For this review, take the finished solid that the model builds, in its own axes (mm). Face numbers are marked on the shaded views. A direction names the side the tool comes from. Give positions to 0.01 mm unless a question says otherwise; leave off trailing zeros. Loops run counter-clockwise (first coordinate to the right, second up) from the corner with the lowest first, then second, coordinate; pieces in that order, holes last. Notation, with made-up numbers: (22, -20) -> (39, -20) arc R30 cw to (39, 17) -> close; hole circle Ø7 at (19, -31). An arc over 180 degrees is marked (long way). Answer as CSV lines item,"result". Start each with the question number.
Item 1: Add section D-D on y = -4. State how many separate pieces and enclosed holes the cut face has, plus the area to 3 significant figures.
Item 2: For L1, parallel to X at y = -6.75, z = -5; L2, parallel to X at y = -6.25, z = -0.75; L3, parallel to Y at x = 24.5, z = 1.5, list the stretches that pass through material, from the lowest coordinate up. Write a range as from..to.
Item 3: Clearance check with flat-ended pins moving along their axes: P1, Ø1.5, axis at x = 28.5, y = -1, coming from the -Z side; P2, Ø1, axis at y = 0, z = -7.5, coming from the -X side; P3, Ø3.5, axis at x = 31.5, y = -2, coming from the -Z side. State where each tip first meets the part, or that it passes through.
Item 4: The part is to be moulded in two halves that separate along Y. For the marked faces 1, 2, 3 and 4, say which applies: +Y half, -Y half, draft (parallel to the pull), parting line (faces both ways), or undercut.
Item 5: Machinability: for the marked faces 5, 6 and 7, which of the approach directions +Z, -Z, +X, -X, +Y, -Y give a long, thin tool a straight path to every point of the face, cutting with its end or side? Answer none if there is none.
Item 6: Add section A-A on x = 29. State the section outline as (y, z) points.
Item 7: Add section C-C on z = -7. State the section outline as (x, y) points.
Item 8: Add section B-B on y = -8.5. State the section outline as (x, z) points, plus the area to 3 significant figures.
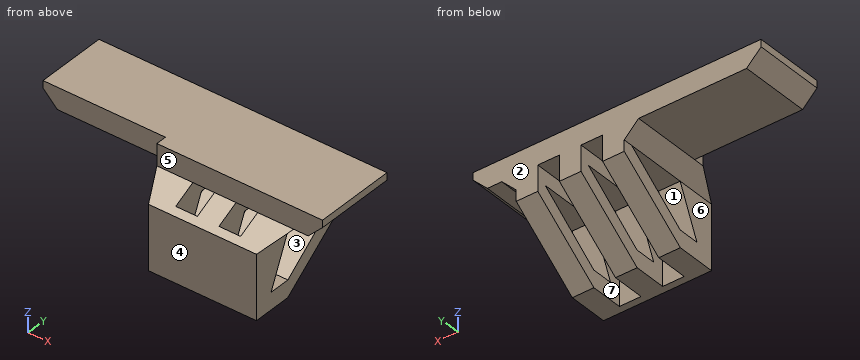
Autodesk Inventor part; units mm, degrees
ref_plane "YZ Plane" through (0, 0, 0) normal (1, 0, 0) x (0, 1, 0)
ref_plane "XZ Plane" through (0, 0, 0) normal (0, 1, 0) x (-1, 0, 0)
ref_plane "XY Plane" through (0, 0, 0) normal (0, 0, 1) x (1, 0, 0)
sketch "Sketch1" plane through (0, 0, 0) normal (0, 0, 1) x (1, 0, 0)
  line L0 (0, 0) -> (5, 0)
  line L1 (5, 0) -> (19, 0)
  line L2 (19, 0) -> (33, 0)
  line L3 (33, 0) -> (28, 0)
  circle A0 centre (5, 0) radius 5
  circle A1 centre (19, 0) radius 5
  circle A2 centre (33, 0) radius 5
  line L4 (0, 0) -> (-1, 0)
  line L5 (38, 0) -> (39, 0)
  line L6 (33, -5) -> (33, -6)
  line L7 (-1, 6) -> (39, 6)
  line L8 (39, 6) -> (39, -6)
  line L9 (39, -6) -> (-1, -6)
  line L10 (-1, -6) -> (-1, 6)
  dimension "d0" = 5
  dimension "d1" = 14
  dimension "d2" = 14
  dimension "d3" = 5
  dimension "d4" = 10
  dimension "d5" = 10
  dimension "d6" = 10
  dimension "d9" = 1
  dimension "d10" = 1
  dimension "d11" = 1
extrude "Extrusion1" add sketch "Sketch1" along normal blind 3
sketch "Sketch2" plane through (-1, 6, 0) normal (0, 1, 0) x (1, 0, 0)
  line L0 (0, -3) -> (40, -3)
  line L1 (19, 2) -> (19, 12)
  line L2 (19, 12) -> (34, 12)
  line L3 (34, 12) -> (34, 2)
  line L4 (34, 0) -> (19, 0)
  line L5 (40, 0) -> (36, 0)
  line L6 (36, 0) -> (34, 2)
  line L7 (0, 0) -> (40, 0)
  line L8 (17, 0) -> (0, 0)
  line L9 (19, 2) -> (17, 0)
  line L10 (36, 0) -> (17, 0)
  point P0 (1, 0)
  dimension "d16" = 12
  dimension "d17" = 2
  dimension "d19" = 2
  dimension "d20" = 2
extrude "Extrusion2" add sketch "Sketch2" against normal blind 16
sketch "Sketch3" plane through (-1, 6, 3) normal (0, 1, 0) x (1, 0, 0)
  line L0 (34, 5) -> (34, 15)
  line L1 (34, 5) -> (34, -8.5215)
  line L2 (34, -8.5215) -> (31, -8.5215)
  line L3 (31, -8.5215) -> (28, -8.5215)
  line L4 (28, -8.5215) -> (25, -8.5215)
  line L5 (25, -8.5215) -> (22, -8.5215)
  line L6 (22, -8.5215) -> (19, -8.5215)
  line L7 (34, 5) -> (34, 3)
  line L8 (17, 3) -> (36, 3)
  line L9 (31, 3) -> (31, 15)
  line L10 (34, 15) -> (19, 15)
  line L11 (31, 15) -> (34, 15)
  line L12 (34, 15) -> (34, 5)
  line L13 (34, 3) -> (31, 3)
  line L14 (31, 3) -> (28, 3)
  line L15 (28, 3) -> (28, 15)
  line L16 (28, 15) -> (31, 15)
  line L17 (28, 3) -> (25, 3)
  line L18 (25, 3) -> (25, 15)
  line L19 (25, 15) -> (28, 15)
  line L20 (25, 3) -> (22, 3)
  line L21 (22, 3) -> (22, 15)
  line L22 (22, 15) -> (25, 15)
  line L23 (22, 3) -> (19, 3)
  line L24 (19, 15) -> (19, 5)
  line L25 (19, 3) -> (19, 15)
  line L26 (19, 15) -> (22, 15)
  point P0 (1, 3)
  dimension "d27" = 3
  dimension "d28" = 3
  dimension "d29" = 3
  dimension "d30" = 3
  dimension "d31" = 3
extrude "Extrusion3" cut sketch "Sketch3" against normal blind 15 contours L9 L8 L15 L10 | L18 L8 L21 L10
sketch "Sketch4" plane through (39, -6, 0) normal (1, 0, 0) x (0, 0, -1)
  line L0 (2, 12) -> (2, -4)
  line L1 (0, 0) -> (2, -4)
  line L2 (2, -4) -> (2, 0)
  line L3 (0, 0) -> (2, 0)
  line L4 (2, 12) -> (2, 10)
  line L5 (12, -3) -> (2, 10)
  line L6 (2, 0) -> (2, 1.5)
  line L7 (2, 10) -> (2, 1.5)
  line L8 (2, 1.5) -> (12, -3)
  line L9 (2, 12) -> (12, 12)
  line L10 (12, 12) -> (12, -4)
  line L11 (12, -3) -> (12, -1)
  line L12 (12, -1) -> (12, 0)
  line L13 (12, 0) -> (3, 12)
  line L14 (2, 12) -> (3, 12)
  line L15 (3, 12) -> (12, 12)
  line L16 (12, 12) -> (12, 0)
  line L17 (0, 0) -> (0, -3)
  line L18 (0, 0) -> (0, -4)
  line L19 (0, 0) -> (0, -4)
  line L20 (2, -4) -> (0, -4)
  line L21 (0, -4) -> (2, -4)
  line L22 (8.5385, 1.5) -> (8.5385, -1.4423)
  point P0 (0, 6)
  dimension "d34" = 2
  dimension "d35" = 1.5
  dimension "d37" = 2
  dimension "d38" = 1
extrude "Extrusion5" cut sketch "Sketch4" against normal blind 25 contours L5 L22 L8 L0 | L9 L10 L13 | L20 L18 L17 L1
chamfer "Chamfer1" distance 2 angle 45 1 edges at (-1, 0, 0)
chamfer "Chamfer2" distance 2 angle 45 1 edges at (39, 0, 0)
sketch "Sketch5" plane through (33, 6, -2) normal (1, 0, 0) x (0, 0, -1)
  line L0 (10, -16) -> (0, -16)
  line L1 (10, -16) -> (8.9, -16)
  line L2 (8.9, -16) -> (8.9, -9)
  line L3 (8.9, -9) -> (10, -9)
  line L4 (10, -9) -> (10, -16)
  point P0 (-2, -6)
  dimension "d49" = 1.1
  dimension "d50" = 7
extrude "Extrusion6" cut sketch "Sketch5" against normal blind 15
sketch "Sketch6" plane through (0, 0, 0) normal (0, 0, -1) x (-1, 0, 0)
  line L0 (-1, -6) -> (-16, -6)
  line L1 (1, 6) -> (1, -6)
  line L2 (-16, -6) -> (1, -6)
  line L3 (1, -6) -> (1, -4.5)
  line L4 (1, -4.5) -> (-16, -4.5)
  line L5 (-16, -4.5) -> (-16, -6)
  point P0 (0, 0)
  dimension "d53" = 1.5
extrude "Extrusion7" cut sketch "Sketch6" against normal blind 10
sketch "Sketch7" plane through (0, 0, 3) normal (0, 0, 1) x (1, 0, 0)
  line L0 (39, 6) -> (-1, 6)
  line L1 (39, -6) -> (39, 6)
  line L2 (-1, 6) -> (39, 6)
  line L3 (39, 6) -> (39, 5.3)
  line L4 (39, 5.3) -> (-1, 5.3)
  line L5 (-1, 5.3) -> (-1, 6)
  point P0 (0, 0)
  dimension "d56" = 0.7
extrude "Extrusion8" cut sketch "Sketch7" against normal blind 10
equation "\"d20\" = d19"
properties part number "StandBtn"
Computed values:
1,separate pieces,"4"
1,enclosed holes,"0"
1,area,"159 mm²"
2,L1,"18..21, 24..27, 30..33"
2,L2,"16.75..21, 24..27, 30..34.25"
2,L3,"-6..5.3"
3,P1,"z = 0"
3,P2,"x = 18"
3,P3,"z = -10.31"
4,face 1,"undercut"
4,face 2,"+Y half"
4,face 3,"undercut"
4,face 4,"-Y half"
5,face 5,"+Z, +X, -X, -Y"
5,face 6,"-Z, -X, +Y, -Y"
5,face 7,"-Z, +Y"
6,outline,"(-10, -10.9) -> (-9, -10.9) -> (-9, -1.5) -> (-10, -2) -> close; (-6, 0) -> (5.3, 0) -> (5.3, 3) -> (-6, 3) -> close"
7,outline,"(18, -10) -> (33, -10) -> (33, -6.75) -> (30, -6.75) -> (30, -9) -> (27, -9) -> (27, -6.75) -> (24, -6.75) -> (24, -9) -> (21, -9) -> (21, -6.75) -> (18, -6.75) -> close; (18, -2.5) -> (21, -2.5) -> (21, 0.67) -> (18, 0.67) -> close; (24, -2.5) -> (27, -2.5) -> (27, 0.67) -> (24, 0.67) -> close; (30, -2.5) -> (33, -2.5) -> (33, 0.67) -> (30, 0.67) -> close"
8,outline,"(17.25, -1.25) -> (18, -2) -> (18, -10.9) -> (21, -10.9) -> (21, -1.25) -> close; (24, -10.9) -> (27, -10.9) -> (27, -1.25) -> (24, -1.25) -> close; (30, -10.9) -> (33, -10.9) -> (33, -2) -> (33.75, -1.25) -> (30, -1.25) -> close"
8,area,"87.4 mm²"
